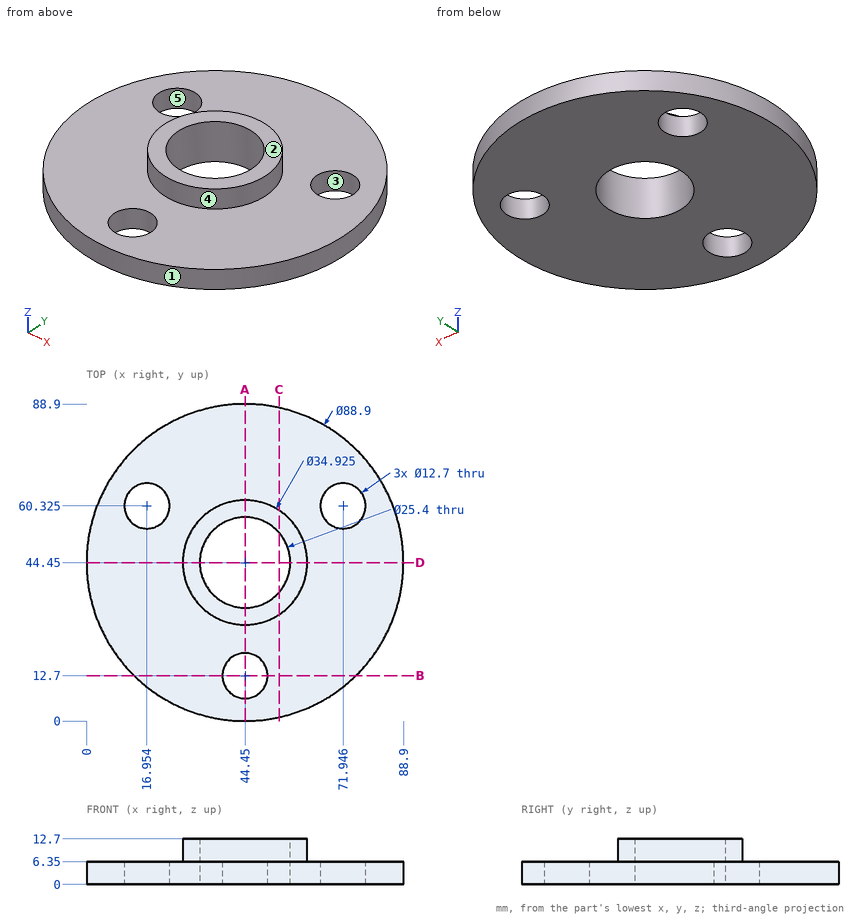
Design review of the part shown in the three views and the two pictorial views. Dimensions are in mm from the part's minimum x, y and z. A direction names the side the tool comes from. Round coordinates to 2 decimals unless told otherwise and drop trailing zeros. Loops run counter-clockwise (first coordinate to the right, second up) from the corner with the lowest first, then second, coordinate; pieces in that order, holes last. Notation, with made-up numbers: M 44.5,-24 L 87.5,-24 A28 ccw 87.5,4 Z; hole C 15.5,68.25 d10. An arc over 180 degrees is marked long. Answer as a JSON object with one key per item and string values.
Item 1: For line 1 along Y through (x, z) = (44.45, 9.5); line 2 along Y through (x, z) = (48.5, 2.5) (1 decimal); line 3 along X through (y, z) = (61, 0.75) (1 decimal), list the stretches that pass through material, from the lowest coordinate up.
Check sheet entries:
{"line 1": "26.99 to 31.75, 57.15 to 61.91", "line 2": "0.2 to 7.8, 17.6 to 32.4, 56.5 to 88.7", "line 3": "3.2 to 10.6, 23.3 to 65.6, 78.3 to 85.7"}
Item 2: Clearance check with flat-ended pins moving along their axes: P1, Ø1, axis at y = 63, z = 1.5, coming from the +X side; P2, Ø5, axis at y = 71.5, z = 11, coming from the +X side; P3, Ø16.5, axis at x = 44.45, y = 12.7, coming from the -Z side; P4, Ø10, axis at x = 47, y = 72, coming from the +Z side. State where each tip first meets the part, or that it passes through.
Check sheet entries:
{"P1": "x = 85.07", "P2": "through", "P3": "z = 0", "P4": "z = 6.35"}
Item 3: We need section D-D, the plane y = 44.45. State the section outline as (x, z) points.
Check sheet entries:
{"outline": "M 0,0 L 31.75,0 L 31.75,12.7 L 26.99,12.7 L 26.99,6.35 L 0,6.35 Z; M 57.15,0 L 88.9,0 L 88.9,6.35 L 61.91,6.35 L 61.91,12.7 L 57.15,12.7 Z"}
Item 4: The part is to be moulded in two halves that separate along Y. For the marked faces 1, 2 and 3, say which applies: +Y half, -Y half, draft (parallel to the pull), parting line (faces both ways), or undercut.
Check sheet entries:
{"face 1": "parting line", "face 2": "draft", "face 3": "undercut"}
Item 5: Tool access review of the marked faces 4 and 5: name each direction out of +Z, -Z, +X, -X, +Y, -Y from which nothing blocks a thin tool from reaching the whole face with its end or side.
Check sheet entries:
{"face 4": "+Z", "face 5": "+Z, -Z"}
Item 6: We need section A-A, the plane x = 44.45. State the section outline as (y, z) points, and give its area (3 significant figures).
Check sheet entries:
{"outline": "M 0,0 L 6.35,0 L 6.35,6.35 L 0,6.35 Z; M 19.05,0 L 31.75,0 L 31.75,12.7 L 26.99,12.7 L 26.99,6.35 L 19.05,6.35 Z; M 57.15,0 L 88.9,0 L 88.9,6.35 L 61.91,6.35 L 61.91,12.7 L 57.15,12.7 Z", "area": "383 mm2"}
Item 7: We need section B-B, the plane y = 12.7. State the section outline as (x, z) points.
Check sheet entries:
{"outline": "M 13.34,0 L 38.1,0 L 38.1,6.35 L 13.34,6.35 Z; M 50.8,0 L 75.56,0 L 75.56,6.35 L 50.8,6.35 Z"}
Item 8: We need section C-C, the plane x = 54. State the section outline as (y, z) points, and give its area (3 significant figures).
Check sheet entries:
{"outline": "M 1.04,0 L 36.08,0 L 36.08,12.7 L 29.83,12.7 L 29.83,6.35 L 1.04,6.35 Z; M 52.82,0 L 87.86,0 L 87.86,6.35 L 59.07,6.35 L 59.07,12.7 L 52.82,12.7 Z", "area": "524 mm2"}
